The figure shows three views and two pictorial views of one solid part (mm, origin at its lowest corner). Answer the questions. Round coordinates to 2 decimals unless told otherwise and drop trailing zeros. Order: outer loops, then holes, each group sorted by start corner. A loop starts at its lowest first (then second) coordinate and runs counter-clockwise, first axis right, second up. Notation, with made-up numbers: (37.5, -25) -> (89.5, -25) arc R20 cw to (89.5, -2) -> close; hole circle Ø6 at (28.5, -18.75). An arc over 180 degrees is marked (long way). Answer in a Markdown table with one row per item. Add a question column.
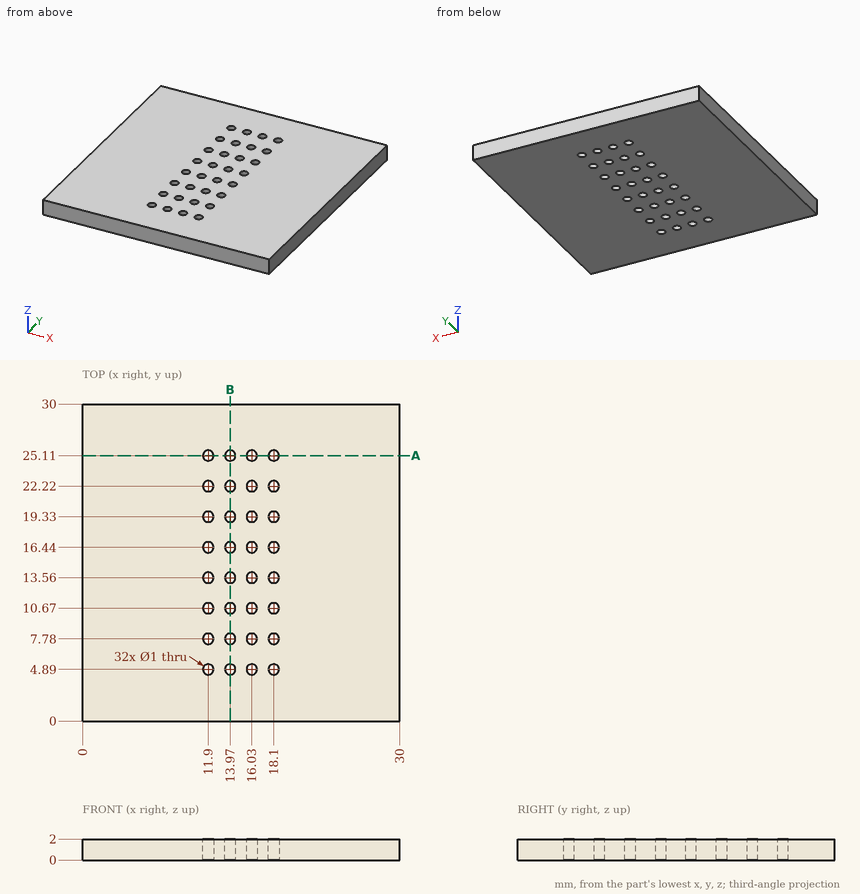
1. The part is cut by section A-A (y = 25.11). Give the vertices of the cut face in (x, z).
2. The part is cut by section B-B (x = 13.97). Give the number of separate pieces and of enclosed holes in the cut face, then the cut area to 3 significant figures.
3. A straight line is drawn through the part: line 1 along X through (y, z) = (19.75, 1.2). Find the intervals that lie inside material, in ascending order.
Report:
| question | item | result |
|---|---|---|
| 1 | outline | (0, 0) -> (11.4, 0) -> (11.4, 2) -> (0, 2) -> close; (12.4, 0) -> (13.47, 0) -> (13.47, 2) -> (12.4, 2) -> close; (14.47, 0) -> (15.53, 0) -> (15.53, 2) -> (14.47, 2) -> close; (16.53, 0) -> (17.6, 0) -> (17.6, 2) -> (16.53, 2) -> close; (18.6, 0) -> (30, 0) -> (30, 2) -> (18.6, 2) -> close |
| 2 | separate pieces | 9 |
| 2 | enclosed holes | 0 |
| 2 | area | 44.0 mm^2 |
| 3 | line 1 | x = 0 to 11.63, 12.17 to 13.7, 14.24 to 15.76, 16.3 to 17.83, 18.37 to 30 |
